Part model, mm, in its own coordinate system. Face numbers are marked on the shaded views. A direction names the side the tool comes from. Give positions to 0.01 mm unless a question says otherwise; leave off trailing zeros. Order: outer loops, then holes, each group sorted by start corner. A loop starts at its lowest first (then second) coordinate and runs counter-clockwise, first axis right, second up. Notation, with made-up numbers: (-38.5, 64.25) -> (-31.5, 64.25) arc R23 ccw to (-31.5, 98.25) -> close; hole circle Ø2 at (-29.5, 46). An arc over 180 degrees is marked (long way). Write item = value, one per line. Start each with the question number.
Item 1: Flat gauge pins, fed straight in: P1, Ø4.5, axis at x = 50, y = 14.5, coming from the +Z side; P2, Ø1.5, axis at x = 87, z = 78, coming from the -Y side; P3, Ø12, axis at x = 60, y = 24.5, coming from the -Z side; P4, Ø10, axis at x = 60.5, z = 68.5, coming from the +Y side. Where does each tip first touch, or does it go through?
Item 2: Drill centre lines: line 1 along Y through (x, z) = (82.5, 87.5); line 2 along X through (y, z) = (-1, 5.5); line 3 along X through (y, z) = (2, 9.5). Where is each one in solid material? Low to high.
Item 3: Band-saw the part on C-C on y = 8. Write the cut outline in (x, z).
Item 4: Band-saw the part on B-B on z = 57. Write the cut outline in (x, y).
Item 5: Tool access for the marked faces 1, 2 and 3: list every direction of +Z, -Z, +X, -X, +Y, -Y with a clear straight run to the whole face (end or side of a thin tool).
```python
from build123d import *

# Parameters (mm, degrees)
F0_W      = 100
F0_H      = 110
F1_DEPTH  = 3
F3_DEPTH  = 25
F4_W      = 15
F4_H      = 6
F5_DEPTH  = 30
F6_R      = 3
F7_R      = 2.99999
F8_R      = 1.5
F9_DEPTH  = 25
F10_R     = 1.5
F11_DEPTH = 25


# Not quite as in the source:
# - a fillet or chamfer is up to 0.001 mm smaller than in the source, because OpenCascade refuses the exact size


with BuildPart() as f1:
    # F0 (on Front) → F1 (new body)
    with BuildSketch(Plane.XZ):
        with Locations((50, 55)):
            Rectangle(F0_W, F0_H)
    extrude(amount=F1_DEPTH)

    # F2 (on face) → F3 (cut)
    with BuildSketch(Plane.XZ.offset(3)):
        with BuildLine():
            Line((0, 110), (0, 65))
            ThreePointArc((0, 65), (16.3054104548, 84.5617848231), (17.5, 110))
            Line((17.5, 110), (0, 110))
        make_face()
        with BuildLine():
            Line((100, 110), (82.5, 110))
            ThreePointArc((82.5, 110), (83.6945895452, 84.5617848231), (100, 65))
            Line((100, 65), (100, 110))
        make_face()
        with BuildLine():
            ThreePointArc((100, 45), (83.6945895452, 25.4382151769), (82.5, 0))
            Line((82.5, 0), (100, 0))
            Line((100, 0), (100, 45))
        make_face()
        with BuildLine():
            Line((0, 45), (0, 0))
            Line((0, 0), (17.5, 0))
            ThreePointArc((17.5, 0), (16.3054104548, 25.4382151769), (0, 45))
        make_face()
    extrude(amount=-F3_DEPTH, mode=Mode.SUBTRACT)

    # F4 (on face) → F5 (join)
    with BuildSketch(Plane(origin=(0, 0, 0), x_dir=(-1, 0, 0), z_dir=(0, 1, 0))):
        with Locations((-50, 7)):
            Rectangle(F4_W, F4_H)
    extrude(amount=F5_DEPTH)

    # F6
    f6_edges = [f1.edges().sort_by_distance(p)[0] for p in [
        (50, 30, 4),
    ]]
    fillet(f6_edges, radius=F6_R)

    # F7 (radius 3 in the source; OpenCascade refuses exactly that, so slightly less here)
    f7_edges = [f1.edges().sort_by_distance(p)[0] for p in [
        (50, 30, 10),
    ]]
    fillet(f7_edges, radius=F7_R)

    # F8 (on face) → F9 (cut)
    with BuildSketch(Plane(origin=(0, 0, 0), x_dir=(-1, 0, 0), z_dir=(0, 1, 0))):
        with Locations((-40.1520836353, 6.8762069568)):
            Circle(F8_R)
        with Locations((-60.1520836353, 6.8762069568)):
            Circle(F8_R)
    extrude(amount=-F9_DEPTH, mode=Mode.SUBTRACT)

    # F10 (on face) → F11 (cut)
    with BuildSketch(Plane.XZ.offset(3)):
        with Locations((23.3403220773, 107.6833680272)):
            Circle(F10_R)
        with Locations((76.8845230341, 107.3717549443)):
            Circle(F10_R)
    extrude(amount=-F11_DEPTH, mode=Mode.SUBTRACT)


solid = f1.part
```
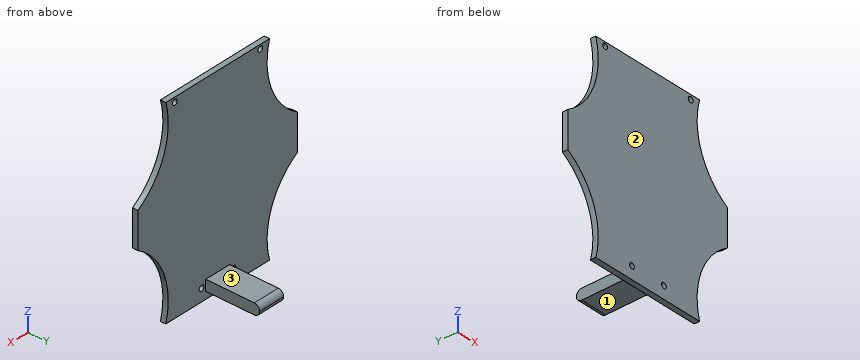
Values found:
q1.P1 = 10
q1.P2 = -3
q1.P3 = 4
q1.P4 = 0
q2.line_1 = -3 to 0
q2.line_2 = 18.65 to 39.56, 40.75 to 59.56, 60.75 to 81.35
q2.line_3 = 42.5 to 57.5
q3.outline = (42.5, 4) -> (57.5, 4) -> (57.5, 10) -> (42.5, 10) -> close
q4.outline = (0, -3) -> (100, -3) -> (100, 0) -> (0, 0) -> close
q5.face_1 = -Z, +X, -X, +Y
q5.face_2 = +Z, -Z, +X, -X, -Y
q5.face_3 = +Z, +X, -X, +Y
